Design review of the part shown in the three views and the two pictorial views. Dimensions are in mm from the part's minimum x, y and z. A direction names the side the tool comes from. Coordinates: 2 decimals unless noted, no trailing zeros. Write each loop counter-clockwise with the first axis right and the second up, starting at its lowest first coordinate (ties: lowest second). Pieces come first, ordered by that corner, then holes. Notation, with made-up numbers: (87.5, 55) -> (105.5, 55) arc R18 ccw to (105.5, 69) -> close; hole circle Ø6 at (63, 75.5). An arc over 180 degrees is marked (long way). Write item = value, one per line. Start each with the question number.
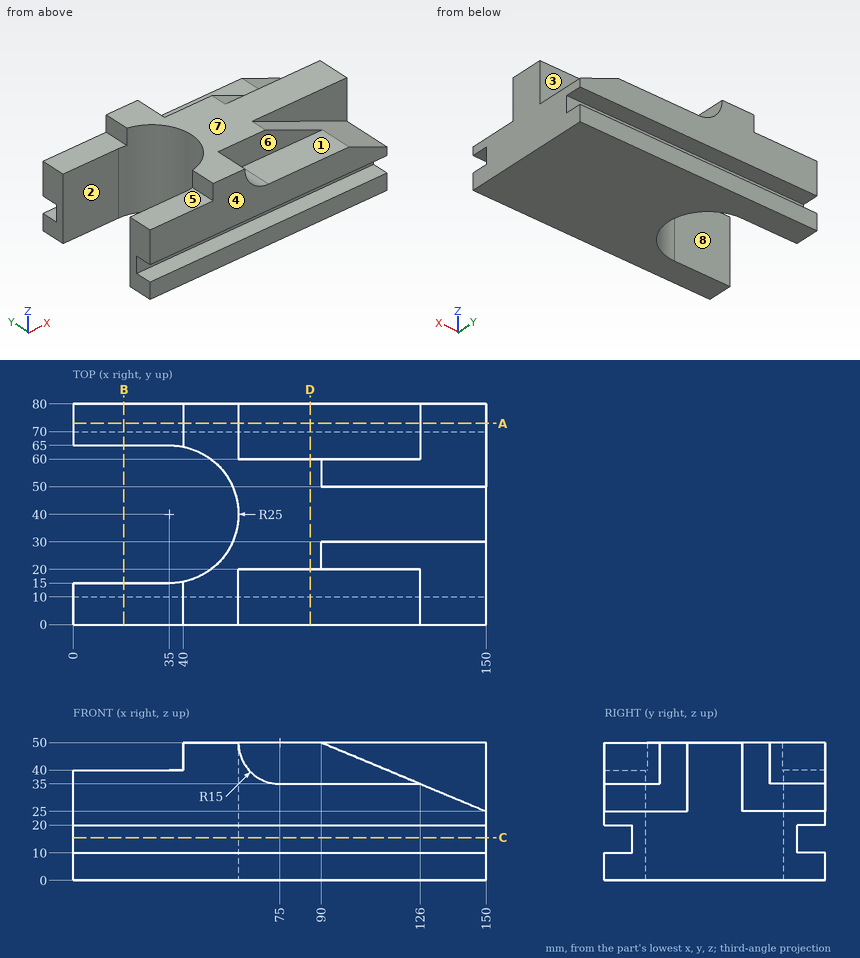
(1) Take a section at A-A, the plane y = 73. State the section outline as (x, z) points, then the cut area to 3 significant figures.
(2) Take a section at D-D, the plane x = 86. State the section outline as (y, z) points.
(3) For pin 1 Ø8 at (x, y) = (78, 74) entering from +Z; pin 2 Ø2 at (x, y) = (128, 53) entering from -Z; pin 3 Ø8 at (y, z) = (73, 45.5) entering from -X; pin 4 Ø5 at (y, z) = (51.5, 45) entering from -X, all flat-tipped, find the tip position at first contact; note any pin that passes through.
(4) Take a section at B-B, the plane x = 18.5. State the section outline as (y, z) points.
(5) Take a section at C-C, the plane z = 15.5. State the section outline as (x, y) points.
(6) For the marked faces 1, 2, 3, 4 and 5, list the 3-axis set-ups (+Z, -Z, +X, -X, +Y, -Y) from which the entire face can be reached by the end or side of a thin tool; tool diameter is ignored.
(7) Mouldability with a two-part tool opening along Y and no side actions: class the marked faces 6, 7 and 8 as pulls with the +Y half, pulls with the -Y half, needs draft (parallel to the pull), parting line crosses it, or undercut.
(8) For line 1 (Y direction, x = 40, z = 5.5); line 2 (Z direction, x = 115.5, y = 4); line 3 (Y direction, x = 15.5, z = 19), list the stretches that pass through material, from the lowest coordinate up.
Report:
q1.outline = (0, 0) -> (150, 0) -> (150, 10) -> (0, 10) -> close; (0, 20) -> (150, 20) -> (150, 25) -> (126, 35) -> (75, 35) arc R15 cw to (60, 50) -> (40, 50) -> (40, 40) -> (0, 40) -> close
q1.area = 4,180 mm2
q2.outline = (0, 0) -> (80, 0) -> (80, 10) -> (70, 10) -> (70, 20) -> (80, 20) -> (80, 35) -> (60, 35) -> (60, 50) -> (20, 50) -> (20, 35) -> (0, 35) -> (0, 20) -> (10, 20) -> (10, 10) -> (0, 10) -> close
q3.pin_1 = 35.03
q3.pin_2 = 0
q3.pin_3 = 40
q3.pin_4 = 55.71
q4.outline = (0, 0) -> (15, 0) -> (15, 40) -> (0, 40) -> (0, 20) -> (10, 20) -> (10, 10) -> (0, 10) -> close; (65, 0) -> (80, 0) -> (80, 10) -> (70, 10) -> (70, 20) -> (80, 20) -> (80, 40) -> (65, 40) -> close
q5.outline = (0, 10) -> (150, 10) -> (150, 70) -> (0, 70) -> (0, 65) -> (35, 65) arc R25 cw to (35, 15) -> (0, 15) -> close
q6.face_1 = +Z, +X, -Y
q6.face_2 = +Z, -Z, -X
q6.face_3 = +Z, +X, +Y
q6.face_4 = +Z, -Z, +X, -X, -Y
q6.face_5 = +Z, -X, +Y, -Y
q7.face_6 = pulls with the -Y half
q7.face_7 = needs draft
q7.face_8 = undercut
q8.line_1 = 0 to 15.51, 64.49 to 80
q8.line_2 = 0 to 10, 20 to 35
q8.line_3 = 10 to 15, 65 to 70
